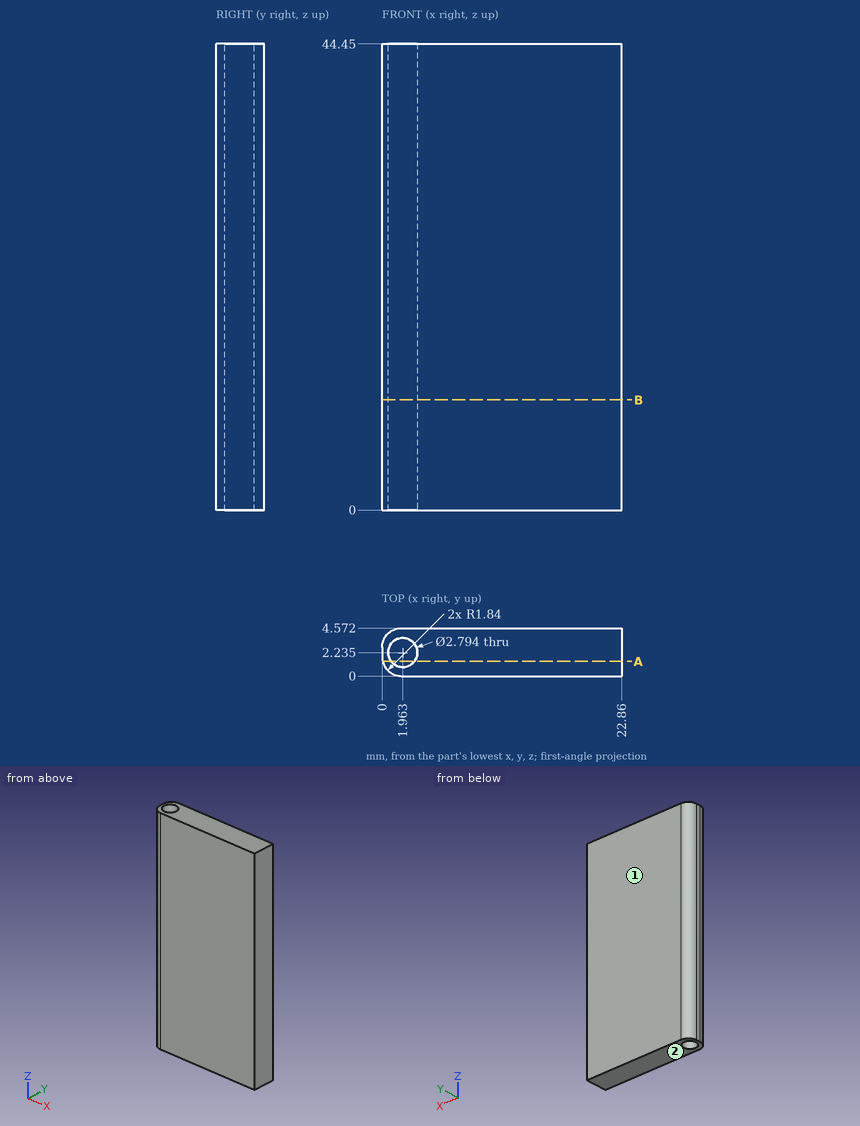
Check sheet for the drawn part. Datum: minimum x, y, z corner. Units: mm. Round coordinates to 2 decimals unless told otherwise and drop trailing zeros. Write each loop counter-clockwise with the first axis right and the second up, starting at its lowest first coordinate (ties: lowest second). Pieces come first, ordered by that corner, then holes. Notation, with made-up numbers: (24, 60.25) -> (82, 60.25) arc R15 cw to (82, 88.25) -> close; hole circle Ø7 at (-3, -26.75). An arc over 180 degrees is marked (long way). Write each question's results on one line, items separated by ' | '.
Q1. Sectioned sample at B-B, the plane z = 10.5. Record the boundary of the cut face in (x, y) (1 decimal).
Derived:
outline: (0, 1.8) arc R1.8 ccw to (1.8, 0) -> (22.9, 0) -> (22.9, 4.6) -> (1.8, 4.6) arc R1.8 ccw to (0, 2.7) -> close; hole circle Ø2.8 at (2, 2.2)
Q2. Thickness scan on probe 1 along X at (y, z) = (1.35, 26.5) (1 decimal); probe 2 along X at (y, z) = (2.7, 8) (1 decimal); probe 3 along X at (y, z) = (3.75, 39). Record the ranges inside material, lowest first.
Derived:
probe 1: x = 0.1 to 0.9, 3 to 22.9 | probe 2: x = 0 to 0.6, 3.3 to 22.9 | probe 3: x = 0.31 to 22.86
Q3. Draft check along Z on the marked faces 1 and 2. Enter one of: released by +Z, released by -Z, zero draft, split by the parting line, or undercut.
Derived:
face 1: zero draft | face 2: released by -Z
Q4. Sectioned sample at A-A, the plane y = 1.4. Record the boundary of the cut face in (x, z).
Derived:
outline: (0.05, 0) -> (0.84, 0) -> (0.84, 44.45) -> (0.05, 44.45) -> close; (3.08, 0) -> (22.86, 0) -> (22.86, 44.45) -> (3.08, 44.45) -> close
Q5. Go/stop test with a flat-tipped pin: pin 1 Ø1.5 at (x, y) = (7, 3) entering from -Z. Record where the tip stops, or that it passes through.
Derived:
pin 1: stops at z = 0
